```python
from build123d import *

# Parameters (mm, degrees)
F0_W     = 57.15
F0_H     = 57.15
F1_DEPTH = 12.7
F2_R     = 4.2164
F3_DEPTH = 12.701
F4_R     = 6.7437
F5_DEPTH = 7.9502
F7_D     = 2.2606


with BuildPart() as f1:
    # F0 (on Top) → F1 (new body)
    with BuildSketch(Plane.XY):
        with Locations((28.575, -28.575)):
            Rectangle(F0_W, F0_H)
    extrude(amount=F1_DEPTH)

    # F2 (on face) → F3 (cut, through all)
    with BuildSketch(Plane.XY.offset(12.7)):
        with Locations((9.525, -9.779)):
            Circle(F2_R)
        with Locations((47.625, -9.779)):
            Circle(F2_R)
    extrude(amount=-F3_DEPTH, mode=Mode.SUBTRACT)

    # F4 (on face) → F5 (cut)
    with BuildSketch(Plane.XY.offset(12.7)):
        with Locations((9.525, -9.779)):
            Circle(F4_R)
        with Locations((47.625, -9.779)):
            Circle(F4_R)
    extrude(amount=-F5_DEPTH, mode=Mode.SUBTRACT)

    # F7 (through all)
    with Locations(Plane.XY.offset(12.7)):
        with Locations((22.225, -7.6454), (22.225, -48.2346)):
            Hole(F7_D / 2)


solid = f1.part
```
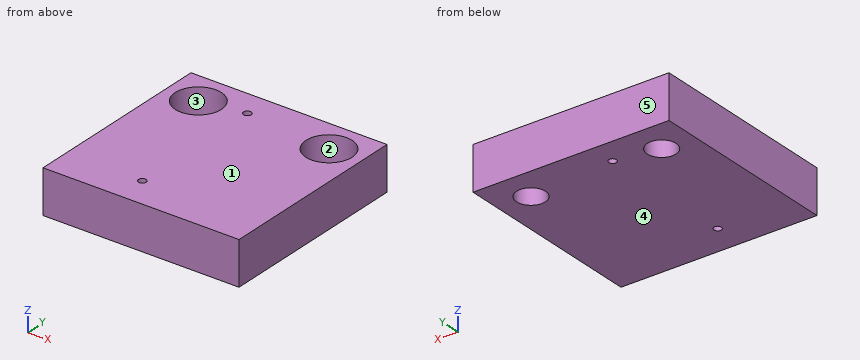
Model file for the job. Use its own axes, mm. Face numbers are marked on the shaded views. A direction names the side the tool comes from. Coordinates: 2 decimals unless noted, no trailing zeros. Loops run counter-clockwise (first coordinate to the right, second up) from the corner with the lowest first, then second, coordinate; pieces in that order, holes last. Notation, with made-up numbers: (69.25, 22) - (79.25, 22) arc R30 cw to (79.25, 60) - close; hole circle Ø6 at (19, 73.25). An arc over 180 degrees is marked (long way). Write item = value, one per line. Start each with the question number.
Item 1: Drop flat-ended pins along their axis: pin 1 Ø7.5 at (x, y) = (47.625, -9.779) entering from -Z; pin 2 Ø2 at (x, y) = (14.5, -8.5) entering from +Z. Give the stop position or say it passes through.
Item 2: Saw through at A-A, the plane x = 44.5. List the corners of the cut face in (y, z), then the cut area to 3 significant figures.
Item 3: Pull direction Y, two halves, no side cores. Call the marked faces 3, 4 and 5: +Y half, -Y half, draft (parallel to the pull), parting line (faces both ways), or undercut.
Item 4: Saw through at C-C, the plane x = 4. List the corners of the cut face in (y, z).
Item 5: Saw through at B-B, the plane z = 3.25. List the corners of the cut face in (x, y) (3 decimals).
Item 6: Wall check: probe 1 along X at (y, z) = (-10, 6); probe 2 along X at (y, z) = (-8, 2.5); probe 3 along X at (y, z) = (-12, 2.5). Give the ranges that are in metal, low to high. Write a range as [from, to].
Item 7: Saw through at D-D, the plane z = 8.5. List the corners of the cut face in (x, y) (3 decimals).
Item 8: 3-axis set-ups, long thin cutter, end or side, ignore diameter. For the marked faces 1 and 2: which of +Z, -Z, +X, -X, +Y, -Y reach the whole face in a straight line?
Answers:
q1.pin_1 = through
q1.pin_2 = 4.75
q2.outline = (-57.15, 0) - (-12.61, 0) - (-12.61, 4.75) - (-15.75, 4.75) - (-15.75, 12.7) - (-57.15, 12.7) - close; (-6.95, 0) - (0, 0) - (0, 12.7) - (-3.8, 12.7) - (-3.8, 4.75) - (-6.95, 4.75) - close
q2.area = 604 mm2
q3.face_3 = undercut
q3.face_4 = draft
q3.face_5 = +Y half
q4.outline = (-57.15, 0) - (0, 0) - (0, 12.7) - (-5.91, 12.7) - (-5.91, 4.75) - (-13.65, 4.75) - (-13.65, 12.7) - (-57.15, 12.7) - close
q5.outline = (0, -57.15) - (57.15, -57.15) - (57.15, 0) - (0, 0) - close; hole circle Ø8.433 at (9.525, -9.779); hole circle Ø2.261 at (22.225, -48.235); hole circle Ø2.261 at (22.225, -7.645); hole circle Ø8.433 at (47.625, -9.779)
q6.probe_1 = [0, 2.78], [16.27, 40.88], [54.37, 57.15]
q6.probe_2 = [0, 5.7], [13.35, 21.15], [23.3, 43.8], [51.45, 57.15]
q6.probe_3 = [0, 5.94], [13.11, 44.04], [51.21, 57.15]
q7.outline = (0, -57.15) - (57.15, -57.15) - (57.15, 0) - (0, 0) - close; hole circle Ø13.487 at (9.525, -9.779); hole circle Ø2.261 at (22.225, -48.235); hole circle Ø2.261 at (22.225, -7.645); hole circle Ø13.487 at (47.625, -9.779)
q8.face_1 = +Z, +X, -X, +Y, -Y
q8.face_2 = +Z
